Geometry check sheet. Reference: the model listing, model coordinates, mm. Round coordinates to 2 decimals unless told otherwise and drop trailing zeros. Write each loop counter-clockwise with the first axis right and the second up, starting at its lowest first coordinate (ties: lowest second). Pieces come first, ordered by that corner, then holes. Notation, with made-up numbers: M 53.25,14 L 61.25,14 A11 cw 61.25,28 Z; hole C 81.25,55.25 d2. An arc over 180 degrees is marked long. Put each result on its own line as item: value. Start each with the question number.
(1) Material ranges on probe 1 along Y at (x, z) = (124, -5.25); probe 2 along Z at (x, y) = (327, -0.25); probe 3 along Z at (x, y) = (95.5, -5.5), recorded low to high.
(2) Section check B-B on y = -2.75. Record the cut outline in (x, z), then the cut area to 3 significant figures.
(3) Section check A-A on x = 489. Record the cut outline in (y, z), then the cut area to 3 significant figures.
(4) Gauge pin test, flat ends, axial feed: pin 1 (3 mm diameter, centred on x = 242.5, z = -4, fed in from +Y); pin 2 (3 mm diameter, centred on x = 166.5, y = 2.5, fed in from +Z); pin 3 (1.5 mm diameter, centred on x = 269.5, y = -2, fed in from +Z). Record the tip position at first contact, or that the pin passes through.
Autodesk Inventor part; units mm, degrees
ref_plane "YZ Plane" through (0, 0, 0) normal (1, 0, 0) x (0, 1, 0)
ref_plane "XZ Plane" through (0, 0, 0) normal (0, 1, 0) x (-1, 0, 0)
ref_plane "XY Plane" through (0, 0, 0) normal (0, 0, 1) x (1, 0, 0)
sketch "Sketch1" plane through (0, 0, 0) normal (1, 0, 0) x (0, 1, 0)
  line L0 (6.35, 3.6662) -> (6.35, -3.6662)
  line L1 (6.35, -3.6662) -> (0, -7.3323)
  line L2 (0, -7.3323) -> (-6.35, -3.6662)
  line L3 (-6.35, -3.6662) -> (-6.35, 3.6662)
  line L4 (-6.35, 3.6662) -> (0, 7.3323)
  line L5 (0, 7.3323) -> (6.35, 3.6662)
  point P0 (0, 0)
  dimension "d0" = 12.7
  dimension "d1" = 12.7
  dimension "d2" = 12.7
  dimension "d3" = 6.35
  dimension "d4" = 120
  dimension "d5" = 120
  dimension "d6" = 6.35
  dimension "d7" = 6.35
extrude "Extrusion1" add sketch "Sketch1" along normal blind 533.4
properties part number "0.5 hex shaft long"
Answers follow:
1. probe 1: y = -3.61 to 3.61
1. probe 2: z = -7.19 to 7.19
1. probe 3: z = -4.16 to 4.16
2. outline: M 0,-5.74 L 533.4,-5.74 L 533.4,5.74 L 0,5.74 Z
2. area: 6,130 mm^2
3. outline: M -6.35,-3.67 L 0,-7.33 L 6.35,-3.67 L 6.35,3.67 L 0,7.33 L -6.35,3.67 Z
3. area: 140 mm^2
4. pin 1: stops at y = 6.35
4. pin 2: stops at z = 6.75
4. pin 3: stops at z = 6.61
